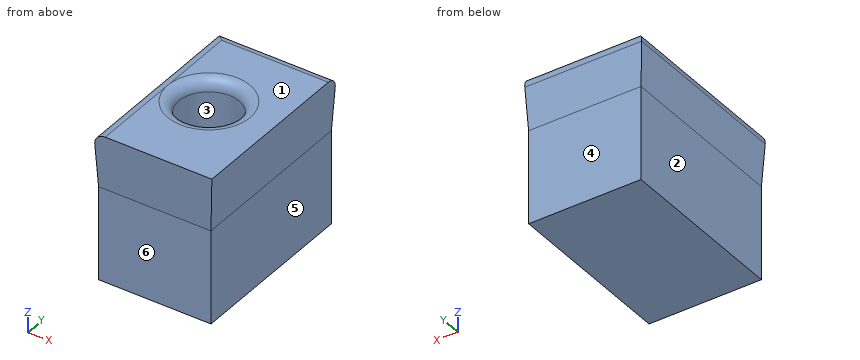
from build123d import *

# Parameters (mm, degrees)
F0_W     = 52.0827807486
F0_H     = 81.0816735029
F1_DEPTH = 43.3417446911
F2_W     = 52.0827807486
F2_H     = 81.0816735029
F2_R     = 15.0408824119
F3_DEPTH = 25.4
F3_TAPER = -3
F4_R     = 5.08
F5_R     = 5.08


with BuildPart() as f1:
    # F0 (on Top) → F1 (new body)
    with BuildSketch(Plane.XY):
        with Locations((-26.0413903743, 40.5408367515)):
            Rectangle(F0_W, F0_H)
    extrude(amount=F1_DEPTH)

    # F2 (on face) → F3 (join)
    with BuildSketch(Plane.XY.offset(43.3417446911)):
        with Locations((-26.0413903743, 40.5408367515)):
            Rectangle(F2_W, F2_H)
        with Locations((-28.9890691638, 40.7522916794)):
            Circle(F2_R, mode=Mode.SUBTRACT)
    extrude(amount=F3_DEPTH, taper=F3_TAPER)

    # F4
    f4_edges = [f1.edges().sort_by_distance(p)[0] for p in [
        (-26.04139, 82.412831, 68.741745),
        (-53.413938, 40.540837, 68.741745),
    ]]
    fillet(f4_edges, radius=F4_R)

    # F5
    f5_edges = [f1.edges().sort_by_distance(p)[0] for p in [
        (-42.698794, 40.752292, 68.741745),
    ]]
    fillet(f5_edges, radius=F5_R)


solid = f1.part
Verification items for the finished model (mm, model axes). Face numbers are marked on the shaded views. A direction names the side the tool comes from. Give positions to 0.01 mm unless a question says otherwise; leave off trailing zeros. Loops run counter-clockwise (first coordinate to the right, second up) from the corner with the lowest first, then second, coordinate; pieces in that order, holes last.
1. Go/stop test with flat-tipped pins: P1, Ø12, axis at y = 12, z = 50, coming from the -X side; P2, Ø13, axis at x = -30.5, z = 24.5, coming from the -Y side; P3, Ø9, axis at x = -33.5, y = 42, coming from the +Z side; P4, Ø3, axis at x = -18, y = 73.5, coming from the -Z side. Record where each tip stops, or that it passes through.
Derived:
P1: stops at x = -52.75
P2: stops at y = 0
P3: stops at z = 43.34
P4: stops at z = 0
2. Material ranges on probe 1 along X at (y, z) = (64, 15); probe 2 along Y at (x, z) = (-46.5, 6); probe 3 along Z at (x, y) = (-27, 51.5), recorded low to high.
Derived:
probe 1: x = -52.08 to 0
probe 2: y = 0 to 81.08
probe 3: z = 0 to 43.34
3. Cross-section at A-A on z = 32. Record the cut outline in (x, y), and give its area (3 significant figures).
Derived:
outline: (-52.08, 0) - (0, 0) - (0, 81.08) - (-52.08, 81.08) - close
area: 4,220 mm2
4. Tool access check on the marked faces 1 and 2. Record the directions out of +Z, -Z, +X, -X, +Y, -Y that give a thin tool (end or side, any length) a straight path to the whole face; none if there is none.
Derived:
face 1: +Z, +X, -X, +Y, -Y
face 2: -Z, -X, +Y, -Y
5. Release check for a two-part mould opening along Y. For the marked faces 3, 4, 5 and 6 record: +Y half, -Y half, draft (parallel to the pull), parting line (faces both ways), or undercut.
Derived:
face 3: undercut
face 4: +Y half
face 5: draft
face 6: -Y half
